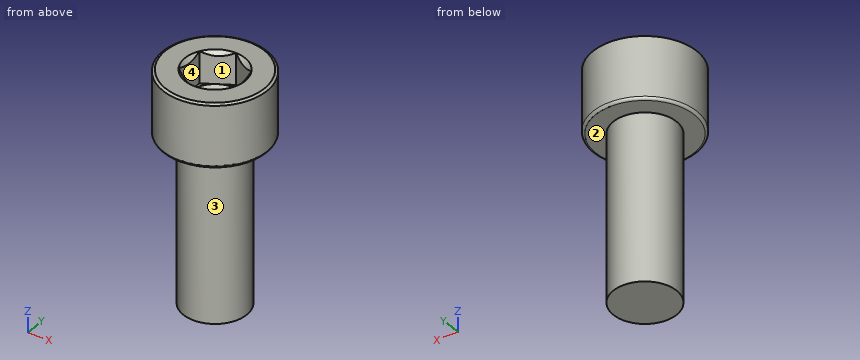
```python
from build123d import *

# Parameters (mm, degrees)
SKETCH1_W          = 12.7
SKETCH1_H          = 2.413
SKETCH4_R          = 3.9624
EXTRUDE1_DEPTH     = 4.826
FILLET1_R          = 0.19304
CHAMFER1_SIZE      = 0.19304
CHAMFER1_SIZE2     = 0.111451696
CUT_EXTRUDE1_DEPTH = 2.413
SKETCH8_R          = 1.984375
CUT_EXTRUDE5_DEPTH = 0.804333333
CUT_EXTRUDE5_DRAFT = -60


with BuildPart() as part:
    # Sketch1 → Revolve1 (revolve)
    with BuildSketch(Plane(origin=(0, 0, 0), x_dir=(0, 0, -1), z_dir=(1, 0, 0))):
        with Locations((6.35, 1.2065)):
            Rectangle(SKETCH1_W, SKETCH1_H)
    revolve(axis=Axis((0, 0, 0), (0, 0, 1)))

    # Sketch4 → Extrude1 (add)
    with BuildSketch(Plane.XY):
        Circle(SKETCH4_R)
    extrude(amount=EXTRUDE1_DEPTH)

    # Fillet1
    fillet1_edges = [part.edges().sort_by_distance(p)[0] for p in [
        (-3.9624, 0, 0),
    ]]
    fillet(fillet1_edges, radius=FILLET1_R)

    # Chamfer1
    chamfer1_edges = [part.edges().sort_by_distance(p)[0] for p in [
        (-3.9624, 0, 4.826),
    ]]
    chamfer1_side = [part.faces().sort_by_distance(p)[0] for p in [
        (0, 0, 4.826),
    ]]
    chamfer(chamfer1_edges, length=CHAMFER1_SIZE, length2=CHAMFER1_SIZE2, reference=chamfer1_side[0])

    # Sketch6 → Cut-Extrude1 (cut)
    with BuildSketch(Plane.XY.offset(4.826)):
        Polygon((0, -2.291358881), (1.984375, -1.14567944), (1.984375, 1.14567944), (0, 2.291358881), (-1.984375, 1.14567944), (-1.984375, -1.14567944), align=None)
    extrude(amount=-CUT_EXTRUDE1_DEPTH, mode=Mode.SUBTRACT)

    # Cut-Extrude4 cone 1 section (through the dimple's axis) → Cut-Extrude4 (revolve, cut)
    with BuildSketch(Plane(origin=(0, 0, 4.826), x_dir=(0, -1, 0), z_dir=(1, 0, 0))):
        Polygon((0, 0), (2.291358881, 0), (0, 2.291358881), align=None)
    revolve(axis=Axis((0, 0, 4.826), (0, 0, -1)), mode=Mode.SUBTRACT)


with BuildPart() as cut_extrude5_tool:
    # Sketch8 → Cut-Extrude5 (with draft: the straight prism first)
    with BuildSketch(Plane.XY.offset(2.413)):
        Circle(SKETCH8_R)
    extrude(amount=-CUT_EXTRUDE5_DEPTH)
    # Cut-Extrude5: the draft: its side faces are tilted about the plane it starts from
    cut_extrude5_sides = [cut_extrude5_tool.faces().sort_by_distance(p)[0] for p in [
        (-1.984375, 0, 2.010833333),
    ]]
    draft(cut_extrude5_sides, Plane.XY.offset(2.413), CUT_EXTRUDE5_DRAFT)


with BuildPart() as part_1:
    add(part.part)

    # Cut-Extrude5: cut by cut_extrude5_tool
    add(cut_extrude5_tool.part, mode=Mode.SUBTRACT)


solid = part_1.part
```
Verification items for the finished model (mm, model axes). Face numbers are marked on the shaded views. Coordinates: 2 decimals unless noted, no trailing zeros. Order: outer loops, then holes, each group sorted by start corner. A loop starts at its lowest first (then second) coordinate and runs counter-clockwise, first axis right, second up. Notation, with made-up numbers: (61, 83.5) -> (67, 83.5) arc R19 cw to (67, 100.5) -> close; hole circle Ø11 at (8.5, -6.5). An arc over 180 degrees is marked (long way). Put each result on its own line as item: value. Start each with the question number.
1) Go/stop test with flat-tipped pins: pin 1 (0.6 mm diameter, centred on x = 0, y = 0, fed in from +Z); pin 2 (3 mm diameter, centred on y = 3, z = -10, fed in from -X); pin 3 (3 mm diameter, centred on y = 2.5, z = 1.5, fed in from +X). Record where each tip stops, or that it passes through.
2) Release check for a two-part mould opening along X. For the marked faces 1, 2, 3 and 4 record: pulls with the +X half, pulls with the -X half, needs draft (parallel to the pull), parting line crosses it, or undercut.
3) Cross-section at A-A (z = -7). Enter the section's corners in (x, y), plus the area to 3 significant figures.
4) Material ranges on L1, parallel to Z at x = -2.75, y = -0.25; L2, parallel to Y at x = 0.75, z = -7.5; L3, parallel to Y at x = 0.25, z = 3.25, recorded low to high.
Geometry check:
1. pin 1: stops at z = 1.61
1. pin 2: stops at x = -1.89
1. pin 3: stops at x = 3.83
2. face 1: undercut
2. face 2: needs draft
2. face 3: parting line crosses it
2. face 4: undercut
3. outline: circle Ø4.83 at (0, 0)
3. area: 18.3 mm^2
4. L1: z = 0 to 4.83
4. L2: y = -2.29 to 2.29
4. L3: y = -3.95 to -2.15, 2.15 to 3.95
